The drawing under review shows one solid part. Ordinate dimensions are in mm from its lowest x, y, z. A direction names the side the tool comes from. Round coordinates to 2 decimals unless told otherwise and drop trailing zeros. Loops run counter-clockwise (first coordinate to the right, second up) from the corner with the lowest first, then second, coordinate; pieces in that order, holes last. Notation, with made-up numbers: M -19.5,78 L 13.5,78 A13 cw 13.5,98 Z; hole C 74,33 d1. An arc over 180 degrees is marked long. Use a Markdown table: item, result.
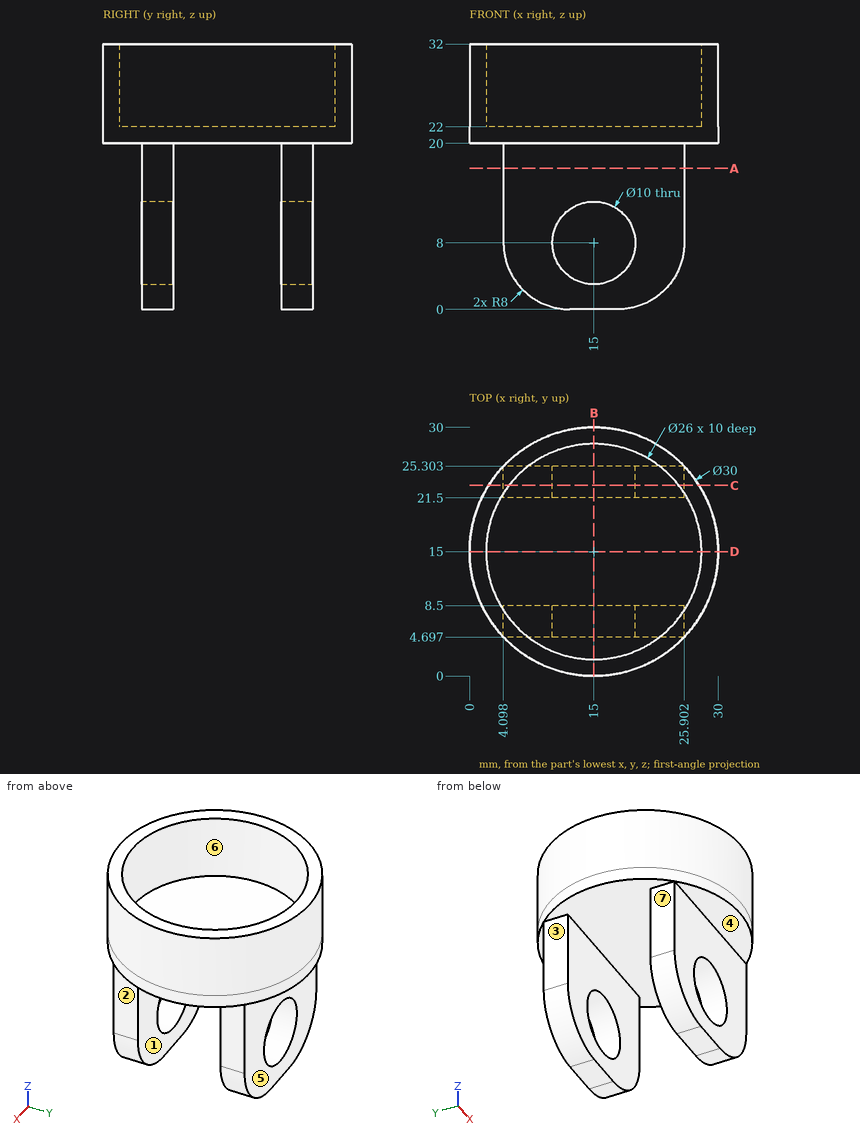
1. Take a section at D-D on y = 15. Give the boundary of the cut face in (x, z), and give its area (3 significant figures).
Check values:
| item | result |
|---|---|
| outline | M 0,20 L 30,20 L 30,32 L 28,32 L 28,22 L 2,22 L 2,32 L 0,32 Z |
| area | 100 mm² |
2. Take a section at C-C on y = 23. Give the boundary of the cut face in (x, z).
Check values:
| item | result |
|---|---|
| outline | M 2.31,20 L 4.1,20 L 4.1,8 A8 ccw 12.1,0 L 17.9,0 A8 ccw 25.9,8 L 25.9,20 L 27.69,20 L 27.69,32 L 25.25,32 L 25.25,22 L 4.75,22 L 4.75,32 L 2.31,32 Z; hole C 15,8 d10 |
3. Machinability: for the marked faces 1, 2, 3 and 4, which of the approach directions +Z, -Z, +X, -X, +Y, -Y give a long, thin tool a straight path to every point of the face, cutting with its end or side? Answer none if there is none.
Check values:
| item | result |
|---|---|
| face 1 | -Z, +X, -X |
| face 2 | -Z, +X, +Y, -Y |
| face 3 | -Z, -X, +Y, -Y |
| face 4 | -Z, +X, -X, -Y |
4. Wall thickness on line 1 along X through (y, z) = (24.25, 8); line 2 along Y through (x, z) = (16.25, 14.5); line 3 along Z through (x, y) = (16, 19.75): over which ranges is each line inside the solid? List them lowest first. Write a range as from..to.
Check values:
| item | result |
|---|---|
| line 1 | x = 4.1..10, 20..25.9 |
| line 2 | y = 4.7..8.5, 21.5..25.3 |
| line 3 | z = 20..22 |
5. Insertion check: pin 1 (8 mm diameter, centred on y = 9, z = 14, fed in from -X); pin 2 (2 mm diameter, centred on x = 25.5, z = 19.5, fed in from +Y); pin 3 (12 mm diameter, centred on y = 8.5, z = 6.5, fed in from +X). Each pin has a flat end and moves straight along its axis. Give the tip position at first contact, or say it passes through.
Check values:
| item | result |
|---|---|
| pin 1 | stops at x = 4.1 |
| pin 2 | stops at y = 26.5 |
| pin 3 | stops at x = 25.9 |
6. The part is to be moulded in two halves that separate along X. For the marked faces 5, 6 and 7, say which applies: pulls with the +X half, pulls with the -X half, needs draft (parallel to the pull), parting line crosses it, or undercut.
Check values:
| item | result |
|---|---|
| face 5 | needs draft |
| face 6 | undercut |
| face 7 | pulls with the -X half |
7. Take a section at A-A on z = 17. Give the boundary of the cut face in (x, y), and give its area (3 significant figures).
Check values:
| item | result |
|---|---|
| outline | M 4.1,4.7 L 25.9,4.7 L 25.9,8.5 L 4.1,8.5 Z; M 4.1,21.5 L 25.9,21.5 L 25.9,25.3 L 4.1,25.3 Z |
| area | 166 mm² |
8. Take a section at B-B on x = 15. Give the boundary of the cut face in (y, z), and give its area (3 significant figures).
Check values:
| item | result |
|---|---|
| outline | M 0,20 L 4.7,20 L 4.7,13 L 8.5,13 L 8.5,20 L 21.5,20 L 21.5,13 L 25.3,13 L 25.3,20 L 30,20 L 30,32 L 28,32 L 28,22 L 2,22 L 2,32 L 0,32 Z; M 4.7,0 L 8.5,0 L 8.5,3 L 4.7,3 Z; M 21.5,0 L 25.3,0 L 25.3,3 L 21.5,3 Z |
| area | 176 mm² |
